Verification items for the finished model (mm, model axes). A direction names the side the tool comes from. Round coordinates to 2 decimals unless told otherwise and drop trailing zeros. Write each loop counter-clockwise with the first axis right and the second up, starting at its lowest first coordinate (ties: lowest second). Pieces come first, ordered by that corner, then holes. Notation, with made-up numbers: (-13, 58.5) -> (0, 58.5) arc R19 cw to (0, 63.5) -> close; hole circle Ø8 at (17.5, 79). An arc over 180 degrees is marked (long way). Answer as a JSON object with one key per item and string values. Group by question number.
(1) Scan lines: L1, parallel to X at y = -12, z = 3.5; L2, parallel to Y at x = 0, z = 23; L3, parallel to Z at x = 3.25, y = -13.5. Record each from-to range of solid material in increasing order. Write a range as from..to.
(2) Sectioned sample at A-A on x = 0. Record the cut outline in (y, z), and give its area (3 significant figures).
(3) Sectioned sample at C-C on z = 3. Record the cut outline in (x, y).
(4) Draft check along Y on faces 1 (the face through (10.5, 0, 2)), 2 (the face through (0.4, 13.6, 3.4)), 3 (the face through (0, 16, 2)). Enter one of: released by +Y, released by -Y, zero draft, split by the parting line, or undercut.
(5) Set-up check for faces 4 (the face through (-7.493, 0.33, 24.72)), 5 (the face through (0.4, -10.4, 3.4)): record each of +Z, -Z, +X, -X, +Y, -Y from which the full face is reachable in a straight line by a thin tool's end or side.
(6) Sectioned sample at D-D on z = 25. Record the cut outline in (x, y), and give its area (3 significant figures).
(7) Sectioned sample at B-B on y = 0. Record the cut outline in (x, z), and give its area (3 significant figures).
(8) Gauge pin test, flat ends, axial feed: pin 1 Ø1 at (x, z) = (-7, 10.5) entering from -Y; pin 2 Ø6 at (x, z) = (3.5, 26.5) entering from -Y; pin 3 Ø5 at (x, z) = (4, 32.5) entering from -Y. Record the tip position at first contact, or that the pin passes through.
```python
from build123d import *

# Parameters (mm, degrees)
F0_R           = 4
F1_DEPTH       = 5
F2_D           = 3.3
F2_DEPTH       = 10
F2_CSINK_D     = 6.72
F2_CSINK_ANGLE = 90
F2_TIP         = 0.9914200214
F3_R           = 7.5
F3_R_2         = 4
F4_DEPTH       = 40


with BuildPart() as f1:
    # F0 (on Top) → F1 (new body)
    with BuildSketch(Plane.XY):
        with BuildLine():
            ThreePointArc((10.5, 12.0726964676), (0, 16), (-10.5, 12.0726964676))
            Line((-10.5, 12.0726964676), (-10.5, -12.0726964676))
            ThreePointArc((-10.5, -12.0726964676), (0, -16), (10.5, -12.0726964676))
            Line((10.5, -12.0726964676), (10.5, 12.0726964676))
        make_face()
        Circle(F0_R, mode=Mode.SUBTRACT)
    extrude(amount=F1_DEPTH)

    # F2
    with Locations(Plane(origin=(0, 0, 0), x_dir=(1, 0, 0), z_dir=(0, 0, -1))):
        with Locations((0, -12), (0, 12)):
            CounterSinkHole(F2_D / 2, F2_CSINK_D / 2, depth=F2_DEPTH, counter_sink_angle=F2_CSINK_ANGLE)
            with Locations((0, 0, -(F2_DEPTH + F2_TIP / 2))):  # 118° drill point
                Cone(0, F2_D / 2, F2_TIP, mode=Mode.SUBTRACT)

    # F3 (on face) → F4 (join)
    with BuildSketch(Plane.XY.offset(5)):
        Circle(F3_R)
        Circle(F3_R_2, mode=Mode.SUBTRACT)
    extrude(amount=F4_DEPTH)


solid = f1.part
```
Computed values:
{
 "1": {"L1": "-10.5..-1.65, 1.65..10.5", "L2": "-7.5..-4, 4..7.5", "L3": "0..5"},
 "2": {"outline": "(-16, 0) -> (-15.36, 0) -> (-13.65, 1.71) -> (-13.65, 5) -> (-16, 5) -> close; (-10.35, 1.71) -> (-8.64, 0) -> (-4, 0) -> (-4, 45) -> (-7.5, 45) -> (-7.5, 5) -> (-10.35, 5) -> close; (4, 0) -> (8.64, 0) -> (10.35, 1.71) -> (10.35, 5) -> (7.5, 5) -> (7.5, 45) -> (4, 45) -> close; (13.65, 1.71) -> (15.36, 0) -> (16, 0) -> (16, 5) -> (13.65, 5) -> close", "area": "361 mm2"},
 "3": {"outline": "(-10.5, -12.07) arc R16 ccw to (10.5, -12.07) -> (10.5, 12.07) arc R16 ccw to (-10.5, 12.07) -> close; hole circle Ø8 at (0, 0); hole circle Ø3.3 at (0, -12); hole circle Ø3.3 at (0, 12)"},
 "4": {"face 1": "zero draft", "face 2": "undercut", "face 3": "released by +Y"},
 "5": {"face 4": "+Z", "face 5": "+Z, -Z"},
 "6": {"outline": "circle Ø15 at (0, 0); hole circle Ø8 at (0, 0)", "area": "126 mm2"},
 "7": {"outline": "(-10.5, 0) -> (-4, 0) -> (-4, 45) -> (-7.5, 45) -> (-7.5, 5) -> (-10.5, 5) -> close; (4, 0) -> (10.5, 0) -> (10.5, 5) -> (7.5, 5) -> (7.5, 45) -> (4, 45) -> close", "area": "345 mm2"},
 "8": {"pin 1": "y = -3.74", "pin 2": "y = -7.48", "pin 3": "y = -7.35"}
}
